Read the model definition and answer for the solid it produces. Units are mm, in the model's axes. Face numbers are marked on the shaded views. A direction names the side the tool comes from. Coordinates: 2 decimals unless noted, no trailing zeros. Order: outer loops, then holes, each group sorted by start corner. A loop starts at its lowest first (then second) coordinate and runs counter-clockwise, first axis right, second up.
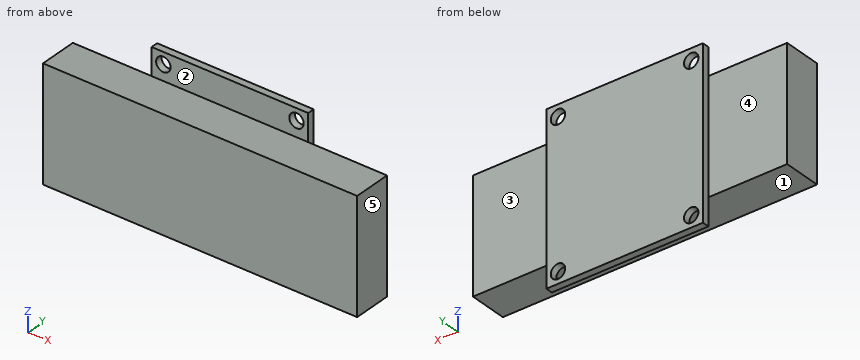
```python
from build123d import *

# Parameters (mm, degrees)
F0_W     = 18.034
F0_H     = 25.908
F0_W_2   = 35.814
F1_DEPTH = 8.7122
F0_H_2   = 6.223
F0_R     = 1.651
F2_DEPTH = 1.6002


with BuildPart() as f1:
    # F0 (on Front) → F1 (new body)
    with BuildSketch(Plane.XZ):
        with Locations((-26.924, 0)):
            Rectangle(F0_W, F0_H)
        Rectangle(F0_W_2, F0_H)
        with Locations((26.924, 0)):
            Rectangle(F0_W, F0_H)
    extrude(amount=F1_DEPTH)

    # F0 (on Front) → F2 (join)
    with BuildSketch(Plane.XZ):
        Rectangle(F0_W_2, F0_H)
        with Locations((0, -16.0655)):
            Rectangle(F0_W_2, F0_H_2)
        with Locations((-15.24, -16.51)):
            Circle(F0_R, mode=Mode.SUBTRACT)
        with Locations((15.24, -16.51)):
            Circle(F0_R, mode=Mode.SUBTRACT)
        with Locations((0, 16.0655)):
            Rectangle(F0_W_2, F0_H_2)
        with Locations((-15.24, 16.51)):
            Circle(F0_R, mode=Mode.SUBTRACT)
        with Locations((15.24, 16.51)):
            Circle(F0_R, mode=Mode.SUBTRACT)
    extrude(amount=-F2_DEPTH)


solid = f1.part
```
1) A cutting plane is placed at D-D, the plane z = -5.5. Determine the outline of the cut face in (x, y).
A:
outline: (-35.94, -8.71) - (35.94, -8.71) - (35.94, 0) - (17.91, 0) - (17.91, 1.6) - (-17.91, 1.6) - (-17.91, 0) - (-35.94, 0) - close
2) Which of the six approach directions +Z, -Z, +X, -X, +Y, -Y give full straight-line access (tool end or side, diameter ignored) to the marked faces 1, 2, 3, 4 and 5?
A:
face 1: -Z, +X, -X, -Y
face 2: +Z, +X, -X, -Y
face 3: +Z, -Z, +X, +Y
face 4: +Z, -Z, -X, +Y
face 5: +Z, -Z, +X, +Y, -Y
3) Straight lines are drawn through the part: line 1 (Z direction, x = 15.24, y = 0.35); line 2 (Y direction, x = 24, z = 6.5); line 3 (Z direction, x = -32, y = -2.75). For each, find the intervals that lie inside material, in ascending order.
A:
line 1: z = -19.18 to -18.16, -14.86 to 14.86, 18.16 to 19.18
line 2: y = -8.71 to 0
line 3: z = -12.95 to 12.95
4) A cutting plane is placed at A-A, the plane z = -16.51. Determine the outline of the cut face in (x, y), and give its area (3 significant figures).
A:
outline: (-17.91, 0) - (-16.89, 0) - (-16.89, 1.6) - (-17.91, 1.6) - close; (-13.59, 0) - (13.59, 0) - (13.59, 1.6) - (-13.59, 1.6) - close; (16.89, 0) - (17.91, 0) - (17.91, 1.6) - (16.89, 1.6) - close
area: 46.7 mm2
5) Flat-ended cylindrical pins translate along their axes: pin 1 Ø0.5 at (y, z) = (1, -2.5) entering from -X; pin 2 Ø5.5 at (x, z) = (-15.24, -16.51) entering from -Y; pin 3 Ø9 at (x, z) = (30.5, 0) entering from +Y; pin 4 Ø4 at (y, z) = (0.5, -1) entering from +X. Find the tip coordinate at first contact, or state that the pin passes through.
A:
pin 1: stops at x = -17.91
pin 2: stops at y = 0
pin 3: stops at y = 0
pin 4: stops at x = 35.94
6) A cutting plane is placed at C-C, the plane y = 0.75. Determine the outline of the cut face in (x, z).
A:
outline: (-17.91, -19.18) - (17.91, -19.18) - (17.91, 19.18) - (-17.91, 19.18) - close; hole circle Ø3.3 at (-15.24, -16.51); hole circle Ø3.3 at (-15.24, 16.51); hole circle Ø3.3 at (15.24, -16.51); hole circle Ø3.3 at (15.24, 16.51)
7) A cutting plane is placed at B-B, the plane x = -15.24. Determine the outline of the cut face in (y, z).
A:
outline: (-8.71, -12.95) - (0, -12.95) - (0, -14.86) - (1.6, -14.86) - (1.6, 14.86) - (0, 14.86) - (0, 12.95) - (-8.71, 12.95) - close; (0, -19.18) - (1.6, -19.18) - (1.6, -18.16) - (0, -18.16) - close; (0, 18.16) - (1.6, 18.16) - (1.6, 19.18) - (0, 19.18) - close
